Verification items for this drawing (mm, ordinates from the low corner). A direction names the side the tool comes from. Round coordinates to 2 decimals unless told otherwise and drop trailing zeros. Loops run counter-clockwise (first coordinate to the right, second up) from the corner with the lowest first, then second, coordinate; pieces in that order, holes last. Notation, with made-up numbers: (-6, 16.25) -> (0, 16.25) arc R27 cw to (0, 37.25) -> close; hole circle Ø5 at (-31.5, 32). An arc over 180 degrees is marked (long way). One line per question, with ' | ' between items.
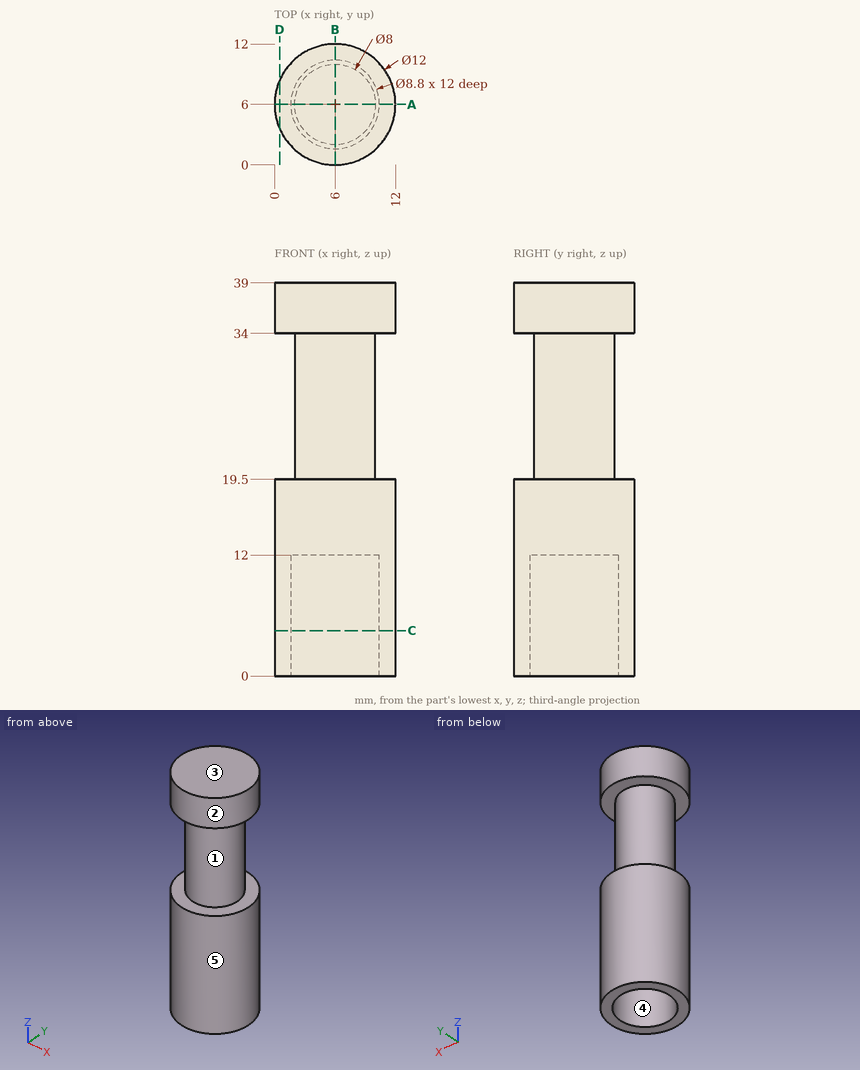
(1) Scan lines: probe 1 along Y at (x, z) = (6, 3.25); probe 2 along Z at (x, y) = (9.5, 2); probe 3 along Z at (x, y) = (9.5, 5.5). Record each from-to range of solid material in increasing order.
Answer:
probe 1: y = 0 to 1.6, 10.4 to 12 | probe 2: z = 0 to 19.5, 34 to 39 | probe 3: z = 12 to 39
(2) Sectioned sample at C-C, the plane z = 4.5. Record the cut outline in (x, y).
Answer:
outline: circle Ø12 at (6, 6); hole circle Ø8.8 at (6, 6)
(3) Go/stop test with flat-tipped pins: pin 1 (1 mm diameter, centred on x = 4, z = 23.5, fed in from -Y); pin 2 (3 mm diameter, centred on x = 7.5, y = 5.5, fed in from -Z); pin 3 (4 mm diameter, centred on x = 2, z = 34.5, fed in from -Y). Record where each tip stops, or that it passes through.
Answer:
pin 1: stops at y = 2.29 | pin 2: stops at z = 12 | pin 3: stops at y = 0.34
(4) Mould release check, pull along Y, two halves, no side actions. Record for the marked faces 3, 4 and 5: +Y half, -Y half, draft (parallel to the pull), parting line (faces both ways), or undercut.
Answer:
face 3: draft | face 4: undercut | face 5: parting line
(5) Sectioned sample at D-D, the plane x = 0.5. Record the cut outline in (y, z), and give its area (3 significant figures).
Answer:
outline: (3.6, 0) -> (8.4, 0) -> (8.4, 19.5) -> (3.6, 19.5) -> close; (3.6, 34) -> (8.4, 34) -> (8.4, 39) -> (3.6, 39) -> close | area: 117 mm2
(6) Set-up check for the marked faces 1 and 2: record each of +Z, -Z, +X, -X, +Y, -Y from which the full face is reachable in a straight line by a thin tool's end or side.
Answer:
face 1: none | face 2: +Z, -Z
(7) Sectioned sample at A-A, the plane y = 6. Record the cut outline in (x, z).
Answer:
outline: (0, 0) -> (1.6, 0) -> (1.6, 12) -> (10.4, 12) -> (10.4, 0) -> (12, 0) -> (12, 19.5) -> (10, 19.5) -> (10, 34) -> (12, 34) -> (12, 39) -> (0, 39) -> (0, 34) -> (2, 34) -> (2, 19.5) -> (0, 19.5) -> close
